from build123d import *

# Parameters (mm, degrees)
SMUSSO1_SIZE             = 0.1
TAGLIO_ESTRUSIONE1_DEPTH = 2


with BuildPart() as part:
    # Schizzo1 → Rivoluzione1 (revolve)
    with BuildSketch(Plane.XY, mode=Mode.PRIVATE) as rivoluzione1_sk:
        Polygon((0, 0), (0, 4), (3.5, 4), (3.5, 0), (2, 0), (2, -12), (0, -12), align=None)
    revolve(rivoluzione1_sk.sketch.rotate(Axis((0, 28.388481997, 0), (0, -1, 0)), 90), axis=Axis((0, 28.388481997, 0), (0, -1, 0)))

    # Smusso1
    smusso1_edges = [part.edges().sort_by_distance(p)[0] for p in [
        (0, -12, -2),
        (0, 4, -3.5),
    ]]
    chamfer(smusso1_edges, length=SMUSSO1_SIZE)

    # Schizzo2 → Taglio-Estrusione1 (cut)
    with BuildSketch(Plane(origin=(0, 4, 0), x_dir=(1, 0, 0), z_dir=(0, 1, 0))):
        Polygon((0, 1.732050808), (-1.5, 0.866025404), (-1.5, -0.866025404), (0, -1.732050808), (1.5, -0.866025404), (1.5, 0.866025404), align=None)
    extrude(amount=-TAGLIO_ESTRUSIONE1_DEPTH, mode=Mode.SUBTRACT)


solid = part.part
Could you check a few things on this model? Use its own coordinates, in mm. A direction names the side the tool comes from. Round coordinates to 2 decimals unless told otherwise and drop trailing zeros. Write each loop counter-clockwise with the first axis right and the second up, starting at its lowest first coordinate (ties: lowest second). Pieces come first, ordered by that corner, then holes. Notation, with made-up numbers: (70.5, -7) - (97.5, -7) arc R9 ccw to (97.5, -3) - close; hole circle Ø1 at (54, 37). An arc over 180 degrees is marked (long way). Put each result on its own line as item: value. Start each with the question number.
(1) I want a section at B-B, the plane y = -2.75. Please give me the cut outline in (x, z), plus the area to 3 significant figures.
(2) I want a section at A-A, the plane z = 0. Please give me the cut outline in (x, y), plus the area to 3 significant figures.
(3) I need wall thicknesses on probe 1 along X at (y, z) = (-4, -1); probe 2 along Y at (x, z) = (0.75, 0.25); probe 3 along Y at (x, z) = (-2, 1.5). Which ranges of each line are inside material? Lowest first, please.
(4) For faces 1 (the flat face through (0.74, 3.014, 1.305)), 2 (the flat face through (-2, 4, 0)), 3 (the flat face through (2, 0, 2)), which set-ups out of +Z, -Z, +X, -X, +Y, -Y let a thin tool reach every point of the face, with its end or its side?
(5) Will these pins go through, and if not, where does the flat tip stop? pin 1 (0.5 mm diameter, centred on y = 2.5, z = -0.5, fed in from +X); pin 2 (1 mm diameter, centred on x = -0.5, z = -2, fed in from -Y).
(6) Thinking about a two-plate mould opening in X: for faces 4 (the flat face through (0, -12, 0)), 5 (the cylindrical face through (3.105, 1.923, 1.615)), 6 (the flat face through (1.5, 3, 0)), which applies, released by +X, released by -X, zero draft, split by the parting line, or undercut?
Here are the results:
1. outline: circle Ø4 at (0, 0)
1. area: 12.6 mm^2
2. outline: (-3.5, 0) - (-2, 0) - (-2, -11.9) - (-1.9, -12) - (1.9, -12) - (2, -11.9) - (2, 0) - (3.5, 0) - (3.5, 3.9) - (3.4, 4) - (1.5, 4) - (1.5, 2) - (-1.5, 2) - (-1.5, 4) - (-3.4, 4) - (-3.5, 3.9) - close
2. area: 70.0 mm^2
3. probe 1: x = -1.73 to 1.73
3. probe 2: y = -12 to 2
3. probe 3: y = 0 to 4
4. face 1: +Y
4. face 2: +Z, -Z, +X, -X, +Y
4. face 3: -Y
5. pin 1: stops at x = 3.49
5. pin 2: stops at y = -12
6. face 4: zero draft
6. face 5: split by the parting line
6. face 6: undercut
